For this review, take the finished solid that the model builds, in its own axes (mm). A direction names the side the tool comes from. Round coordinates to 2 decimals unless told otherwise and drop trailing zeros. Loops run counter-clockwise (first coordinate to the right, second up) from the corner with the lowest first, then second, coordinate; pieces in that order, holes last. Notation, with made-up numbers: (41.5, 75.5) -> (94.5, 75.5) arc R31 cw to (94.5, 103.5) -> close; hole circle Ø8 at (53.25, 65). An arc over 180 degrees is marked (long way). One line per question, with ' | ' between items. Start each with the question number.
1. Consider section C-C (y = -5). Write out the cut boundary in (x, z), and give its area (3 significant figures).
2. For pin 1 Ø4 at (y, z) = (-5, 0) entering from -X; pin 2 Ø2.5 at (y, z) = (-5, 0) entering from -X, all flat-tipped, find the tip position at first contact; note any pin that passes through.
3. Consider section B-B (z = 0). Write out the cut boundary in (x, y), and give its area (3 significant figures).
4. Draft analysis for pull direction Y (two halves, no side actions). For faces 4 (the face through (62.6, -6.2, -0.9)), 5 (the face through (-1, -10, 0)), 6 (the face through (72.5, -3, 0)), state which applies: pulls with the +Y half, pulls with the -Y half, needs draft (parallel to the pull), parting line crosses it, or undercut.
5. For faces 1 (the face through (52.5, -5, 0)), 2 (the face through (-62.64, -6.386, -0.575)), 3 (the face through (-1, -5, -15)), list the 3-axis set-ups (+Z, -Z, +X, -X, +Y, -Y) from which the entire face can be reached by the end or side of a thin tool; tool diameter is ignored.
6. Wall thickness on line 1 along Z through (x, y) = (-59.25, -5): over which ranges is the line inside the solid? List them lowest first.
7. Consider section A-A (x = -61). Write out the cut boundary in (y, z), and give its area (3 significant figures).
```python
from build123d import *

# Parameters (mm, degrees)
F0_W     = 145
F0_H     = 30
F1_DEPTH = 10
F2_R     = 1.5
F3_DEPTH = 20
F4_R     = 1.5
F5_DEPTH = 20


with BuildPart() as f1:
    # F0 (on Front) → F1 (new body)
    with BuildSketch(Plane.XZ):
        Rectangle(F0_W, F0_H)
    extrude(amount=F1_DEPTH)

    # F2 (on face) → F3 (cut)
    with BuildSketch(Plane(origin=(-72.5, 0, 0), x_dir=(0, -1, 0), z_dir=(-1, 0, 0))):
        with Locations((5, 0)):
            Circle(F2_R)
    extrude(amount=-F3_DEPTH, mode=Mode.SUBTRACT)

    # F4 (on face) → F5 (cut)
    with BuildSketch(Plane.YZ.offset(72.5)):
        with Locations((-5, 0)):
            Circle(F4_R)
    extrude(amount=-F5_DEPTH, mode=Mode.SUBTRACT)


solid = f1.part
```
Answer block:
1) outline: (-72.5, -15) -> (72.5, -15) -> (72.5, -1.5) -> (52.5, -1.5) -> (52.5, 1.5) -> (72.5, 1.5) -> (72.5, 15) -> (-72.5, 15) -> (-72.5, 1.5) -> (-52.5, 1.5) -> (-52.5, -1.5) -> (-72.5, -1.5) -> close | area: 4,230 mm2
2) pin 1: stops at x = -72.5 | pin 2: stops at x = -52.5
3) outline: (-72.5, -10) -> (72.5, -10) -> (72.5, -6.5) -> (52.5, -6.5) -> (52.5, -3.5) -> (72.5, -3.5) -> (72.5, 0) -> (-72.5, 0) -> (-72.5, -3.5) -> (-52.5, -3.5) -> (-52.5, -6.5) -> (-72.5, -6.5) -> close | area: 1,330 mm2
4) face 4: undercut | face 5: pulls with the -Y half | face 6: needs draft
5) face 1: +X | face 2: -X | face 3: -Z, +X, -X, +Y, -Y
6) line 1: z = -15 to -1.5, 1.5 to 15
7) outline: (-10, -15) -> (0, -15) -> (0, 15) -> (-10, 15) -> close; hole circle Ø3 at (-5, 0) | area: 293 mm2
